from build123d import *

# Parameters (mm, degrees)
SKETCH1_W                      = 53.9242
SKETCH1_H                      = 44.45
BASE_FLANGE2_DEPTH             = 2.286
EDGE_FLANGE1_STRIP_W           = 10.6172
EDGE_FLANGE1_STRIP_H           = 2.286
EDGE_FLANGE1_STRIP_CUT_DEPTH   = 44.45
EDGE_FLANGE1_STRIP_2_W         = 10.6172
EDGE_FLANGE1_STRIP_2_H         = 2.286
EDGE_FLANGE1_STRIP_CUT_2_DEPTH = 44.45
EDGE_FLANGE1_DEPTH             = 44.45
EDGE_FLANGE1_BEND_DEPTH        = 44.45


# Sheet-metal steps are written as plain solids
with BuildPart() as part:
    # Sketch1 → Base-Flange2 (new body)
    with BuildSketch(Plane(origin=(0, 0, 0), x_dir=(1, 0, 0), z_dir=(0, 1, 0))):
        Rectangle(SKETCH1_W, SKETCH1_H)
    extrude(amount=-BASE_FLANGE2_DEPTH)

    # Edge-Flange1 strip (across the edge) → Edge-Flange1 strip cut (cut)
    with BuildSketch(Plane(origin=(-26.9621, 0, -22.225), x_dir=(1, 0, 0), z_dir=(0, 0, 1))):
        with Locations((-2.286, -1.143)):
            Rectangle(EDGE_FLANGE1_STRIP_W, EDGE_FLANGE1_STRIP_H)
    extrude(amount=EDGE_FLANGE1_STRIP_CUT_DEPTH, mode=Mode.SUBTRACT)

    # Edge-Flange1 strip 2 (across the edge) → Edge-Flange1 strip cut 2 (cut)
    with BuildSketch(Plane(origin=(26.9621, 0, 22.225), x_dir=(-1, 0, 0), z_dir=(0, 0, -1))):
        with Locations((-2.286, -1.143)):
            Rectangle(EDGE_FLANGE1_STRIP_2_W, EDGE_FLANGE1_STRIP_2_H)
    extrude(amount=EDGE_FLANGE1_STRIP_CUT_2_DEPTH, mode=Mode.SUBTRACT)

    # Edge-Flange1 section (across the edge) → Edge-Flange1 (add)
    with BuildSketch(Plane(origin=(-26.9621, 0, -22.225), x_dir=(1, 0, 0), z_dir=(0, 0, 1))):
        with BuildLine():
            Line((0, 0.7366), (0, 13.589))
            Line((0, 13.589), (2.286, 13.589))
            Line((2.286, 13.589), (2.286, 0.7366))
            ThreePointArc((2.286, 0.7366), (2.501745145, 0.215745145), (3.0226, 0))
            Line((3.0226, 0), (3.0226, -2.286))
            ThreePointArc((3.0226, -2.286), (0.885299043, -1.400700957), (0, 0.7366))
        make_face()
    extrude(amount=EDGE_FLANGE1_DEPTH)

    # Edge-Flange1 section 2 (across the edge) → Edge-Flange1 bend (add)
    with BuildSketch(Plane(origin=(26.9621, 0, 22.225), x_dir=(-1, 0, 0), z_dir=(0, 0, -1))):
        with BuildLine():
            Line((0, 0.7366), (0, 13.589))
            Line((0, 13.589), (2.286, 13.589))
            Line((2.286, 13.589), (2.286, 0.7366))
            ThreePointArc((2.286, 0.7366), (2.501745145, 0.215745145), (3.0226, 0))
            Line((3.0226, 0), (3.0226, -2.286))
            ThreePointArc((3.0226, -2.286), (0.885299043, -1.400700957), (0, 0.7366))
        make_face()
    extrude(amount=EDGE_FLANGE1_BEND_DEPTH)


solid = part.part
Verification items for the finished model (mm, model axes). A direction names the side the tool comes from. Coordinates: 2 decimals unless noted, no trailing zeros. Order: outer loops, then holes, each group sorted by start corner. A loop starts at its lowest first (then second) coordinate and runs counter-clockwise, first axis right, second up. Notation, with made-up numbers: M -15,68.5 L 9,68.5 A14 cw 9,76.5 Z; hole C 12,45.5 d6. An arc over 180 degrees is marked long. Return JSON: item names as keys, results as strings.
1) Gauge pin test, flat ends, axial feed: pin 1 (2 mm diameter, centred on x = -3.5, y = 2, fed in from +Z); pin 2 (1 mm diameter, centred on x = 12, z = -6, fed in from +Y). Record the tip position at first contact, or that the pin passes through.
Answer list:
{"pin 1": "through", "pin 2": "y = 0"}
2) Cross-section at A-A, the plane y = 10.25. Record the boundary of the cut face in (x, z) (3 decimals), and give its area (3 significant figures).
Answer list:
{"outline": "M -26.962,-22.225 L -24.676,-22.225 L -24.676,22.225 L -26.962,22.225 Z; M 24.676,-22.225 L 26.962,-22.225 L 26.962,22.225 L 24.676,22.225 Z", "area": "203 mm2"}
3) Cross-section at C-C, the plane x = 18.5. Record the boundary of the cut face in (y, z) (3 decimals), and give its area (3 significant figures).
Answer list:
{"outline": "M -2.286,-22.225 L 0,-22.225 L 0,22.225 L -2.286,22.225 Z", "area": "102 mm2"}
4) Cross-section at B-B, the plane z = -14. Record the boundary of the cut face in (x, y), and give its area (3 significant figures).
Answer list:
{"outline": "M -26.96,0.74 A3.02 ccw -23.94,-2.29 L 23.94,-2.29 A3.02 ccw 26.96,0.74 L 26.96,13.59 L 24.68,13.59 L 24.68,0.74 A0.74 cw 23.94,0 L -23.94,0 A0.74 cw -24.68,0.74 L -24.68,13.59 L -26.96,13.59 Z", "area": "182 mm2"}
5) Thickness scan on L1, parallel to X at y = 9.25, z = -6; L2, parallel to Y at x = -15, z = 9.5; L3, parallel to X at y = 0.5, z = 14. Record the ranges inside material, lowest first. Write a range as [from, to].
Answer list:
{"L1": "[-26.96, -24.68], [24.68, 26.96]", "L2": "[-2.29, 0]", "L3": "[-26.95, -24.64], [24.64, 26.95]"}
6) Access from +Z, -Z, +X, -X, +Y, -Y to the whole of each face (thin tool, end or side, straight path). Record for faces 4 (the flat face through (24.676, 7, 0)), 5 (the flat face through (-26.962, 7, 0)).
Answer list:
{"face 4": "+Z, -Z, +Y", "face 5": "+Z, -Z, -X, +Y, -Y"}
7) Release check for a two-part mould opening along X. For faces 1 (the cylindrical face through (-26.053, -1.424, -0.311)), 2 (the flat face through (-24.676, 7, 0)), 3 (the flat face through (0, -1, 22.225)) record: +X half, -X half, draft (parallel to the pull), parting line (faces both ways), or undercut.
Answer list:
{"face 1": "-X half", "face 2": "undercut", "face 3": "draft"}
